For this review, take the finished solid that the model builds, in its own axes (mm). A direction names the side the tool comes from. Round coordinates to 2 decimals unless told otherwise and drop trailing zeros. Write each loop counter-clockwise with the first axis right and the second up, starting at its lowest first coordinate (ties: lowest second). Pieces come first, ordered by that corner, then holes. Notation, with made-up numbers: M 1,-11.5 L 21,-11.5 A20 ccw 21,18.5 Z; hole C 41.25,6.5 d11. An arc over 180 degrees is marked long. Answer in a Markdown table with one row per item.
```python
from build123d import *

# Parameters (mm, degrees)
SKETCH1_W           = 70
SKETCH1_H           = 120
BOSS_EXTRUDE1_DEPTH = 4
SKETCH2_W           = 34
SKETCH2_H           = 50
BOSS_EXTRUDE2_DEPTH = 50
SKETCH3_R           = 11.1
CUT_EXTRUDE1_DEPTH  = 7
SKETCH5_R           = 7
CUT_EXTRUDE3_DEPTH  = 103.396288995
SKETCH6_R           = 11.05
CUT_EXTRUDE4_DEPTH  = 7
SKETCH7_R           = 12
CUT_EXTRUDE5_DEPTH  = 1.5
SKETCH8_R           = 1.65
BOSS_EXTRUDE3_DEPTH = 6
FILLET1_R           = 3
FILLET2_R           = 6


with BuildPart() as part:
    # Sketch1 → Boss-Extrude1 (new body)
    with BuildSketch(Plane(origin=(0, 0, 0), x_dir=(0, 1, 0), z_dir=(0, 0, 1))):
        Rectangle(SKETCH1_W, SKETCH1_H)
    extrude(amount=BOSS_EXTRUDE1_DEPTH)

    # Sketch2 → Boss-Extrude2 (add)
    with BuildSketch(Plane.XY.offset(4)):
        with Locations((0, -10)):
            Rectangle(SKETCH2_W, SKETCH2_H)
    extrude(amount=BOSS_EXTRUDE2_DEPTH)

    # Sketch3 → Cut-Extrude1 (cut)
    with BuildSketch(Plane.XZ.offset(35)):
        with Locations((0, 34)):
            Circle(SKETCH3_R)
    extrude(amount=-CUT_EXTRUDE1_DEPTH, mode=Mode.SUBTRACT)

    # Sketch5 → Cut-Extrude3 (cut, through all)
    with BuildSketch(Plane.XZ.offset(28)):
        with Locations((0, 34)):
            Circle(SKETCH5_R)
    extrude(amount=-CUT_EXTRUDE3_DEPTH, mode=Mode.SUBTRACT)

    # Sketch6 → Cut-Extrude4 (cut)
    with BuildSketch(Plane(origin=(0, 15, 0), x_dir=(-1, 0, 0), z_dir=(0, 1, 0))):
        with Locations((0, 34)):
            Circle(SKETCH6_R)
    extrude(amount=-CUT_EXTRUDE4_DEPTH, mode=Mode.SUBTRACT)

    # Sketch7 → Cut-Extrude5 (cut)
    with BuildSketch(Plane.XY.offset(4)):
        with Locations((-44, 2.5)):
            Circle(SKETCH7_R)
    extrude(amount=-CUT_EXTRUDE5_DEPTH, mode=Mode.SUBTRACT)

    # Sketch8 → Boss-Extrude3 (add)
    with BuildSketch(Plane(origin=(0, 15, 0), x_dir=(-1, 0, 0), z_dir=(0, 1, 0))):
        Polygon((-17, 4), (-27, 4), (-27, 61), (27, 61), (27, 4), (17, 4), (17, 54), (-17, 54), align=None)
        with Locations(Location((-21.213203436, 55.213203436, 0), (0, 0, 90))):
            Circle(SKETCH8_R, mode=Mode.SUBTRACT)
        with Locations(Location((21.213203436, 55.213203436, 0), (0, 0, 90))):
            Circle(SKETCH8_R, mode=Mode.SUBTRACT)
        with Locations(Location((-21.213203436, 12.786796564, 0), (0, 0, 90))):
            Circle(SKETCH8_R, mode=Mode.SUBTRACT)
        with Locations(Location((21.213203436, 12.786796564, 0), (0, 0, 90))):
            Circle(SKETCH8_R, mode=Mode.SUBTRACT)
    extrude(amount=-BOSS_EXTRUDE3_DEPTH)

    # Fillet1
    fillet1_edges = [part.edges().sort_by_distance(p)[0] for p in [
        (17, -13, 54),
        (-17, -13, 54),
        (27, 12, 4),
        (27, 12, 61),
        (-27, 12, 61),
        (-27, 12, 4),
    ]]
    fillet(fillet1_edges, radius=FILLET1_R)

    # Fillet2
    fillet2_edges = [part.edges().sort_by_distance(p)[0] for p in [
        (17, -13, 4),
        (-17, -13, 4),
    ]]
    fillet(fillet2_edges, radius=FILLET2_R)


solid = part.part
```
Q1. Take a section at C-C (z = 19). State the section outline as (x, y) points, then the cut area to 3 significant figures.
Found:
| item | result |
|---|---|
| outline | M -27,9 L -17,9 L -17,-35 L 17,-35 L 17,9 L 27,9 L 27,15 L -27,15 Z |
| area | 1,820 mm² |
Q2. Insertion check: P1, Ø8, axis at y = 18, z = 20.5, coming from the -X side; P2, Ø1.5, axis at x = 36, y = -12.5, coming from the +Z side; P3, Ø5.5, axis at x = -21.21, z = 55.21, coming from the +Y side; P4, Ø6.5, axis at x = -1, z = 36, coming from the -Y side. Each pin has a flat end and moves straight along its axis. Give the tip position at first contact, or say it passes through.
Found:
| item | result |
|---|---|
| P1 | x = -27 |
| P2 | z = 4 |
| P3 | y = 15 |
| P4 | through |
Q3. Take a section at D-D (x = 44.5). State the section outline as (y, z) points.
Found:
| item | result |
|---|---|
| outline | M -35,0 L 35,0 L 35,4 L -35,4 Z |
Q4. For probe 1 along Y at (x, z) = (-4.5, 20); probe 2 along Z at (x, y) = (0, 11.75); probe 3 along Z at (x, y) = (-12, 16.5), list the stretches that pass through material, from the lowest coordinate up.
Found:
| item | result |
|---|---|
| probe 1 | -35 to 15 |
| probe 2 | 0 to 22.95, 45.05 to 61 |
| probe 3 | 0 to 4 |
Q5. Machinability: for faces 4 (the face through (13, 15, 33)), 5 (the face through (17, -13, 30)), 6 (the face through (-18.711, -12.692, 5.804)), 7 (the face through (-0.2, -28, 26.8)), which of the approach directions +Z, -Z, +X, -X, +Y, -Y give a long, thin tool a straight path to every point of the face, cutting with its end or side? Answer none if there is none.
Found:
| item | result |
|---|---|
| face 4 | +Z, +X, -X, +Y |
| face 5 | +Z, +X, -Y |
| face 6 | +Z, -X, -Y |
| face 7 | -Y |
Q6. Take a section at B-B (y = 2.5). State the section outline as (x, z) points.
Found:
| item | result |
|---|---|
| outline | M -60,0 L 60,0 L 60,4 L 23,4 A6 cw 17,10 L 17,51 A3 ccw 14,54 L -14,54 A3 ccw -17,51 L -17,10 A6 cw -23,4 L -32,4 L -32,2.5 L -56,2.5 L -56,4 L -60,4 Z; hole C 0,34 d14 |
Q7. Take a section at A-A (z = 34). State the section outline as (x, y) points, then the cut area to 3 significant figures.
Found:
| item | result |
|---|---|
| outline | M -27,9 L -17,9 L -17,-35 L -11.1,-35 L -11.1,-28 L -7,-28 L -7,8 L -11.05,8 L -11.05,15 L -27,15 Z; M 7,-28 L 11.1,-28 L 11.1,-35 L 17,-35 L 17,9 L 27,9 L 27,15 L 11.05,15 L 11.05,8 L 7,8 Z |
| area | 1,010 mm² |
Q8. Mouldability with a two-part tool opening along X and no side actions: class faces 1 (the face through (-60, 0, 2)), 2 (the face through (18.804, -12.692, 5.711)), 3 (the face through (-19.82, 12.04, 13.67)) as +X half, -X half, draft (parallel to the pull), parting line (faces both ways), or undercut.
Found:
| item | result |
|---|---|
| face 1 | -X half |
| face 2 | +X half |
| face 3 | undercut |
